The figure shows three views and two pictorial views of one solid part (mm, origin at its lowest corner). Answer the questions. A direction names the side the tool comes from. Round coordinates to 2 decimals unless told otherwise and drop trailing zeros.
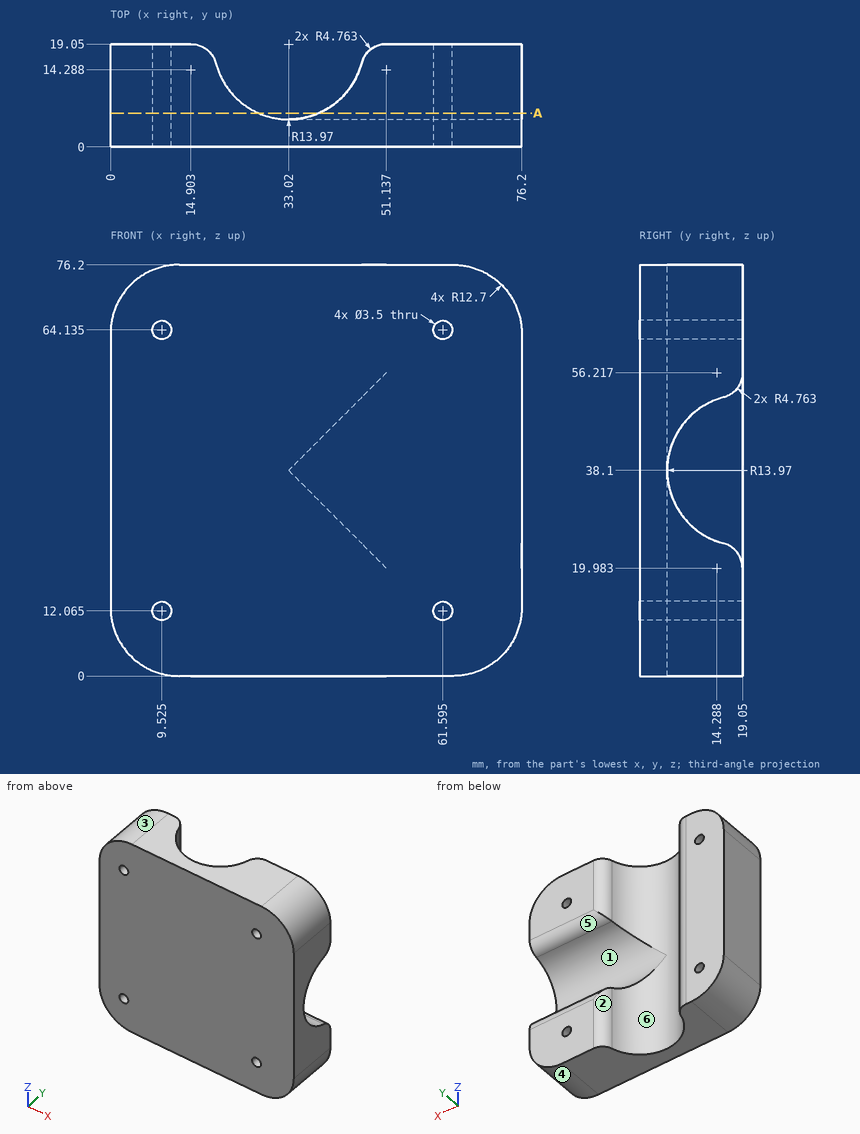
Item 1: Find the intervals of material crossed by line 1 along Z through (x, y) = (63, 17) (1 decimal); line 2 along X through (y, z) = (16, 11) (1 decimal); line 3 along X through (y, z) = (15, 56.5), in increasing order.
Item 2: Find section A-A (y = 6.25). State how many separate pieces and enclosed holes the cut face has, plus the area to 3 significant figures.
Item 3: A tool of negligible diameter and unlimited length cuts with its end or side. For the marked faces 1, 2 and 3, from which of +Z, -Z, +X, -X, +Y, -Y can it reach the whole face along a straight path? Write none if from no direction.
Item 4: Given pin 1 (2 mm diameter, centred on y = 4.5, z = 61, fed in from -X); pin 2 (2 mm diameter, centred on x = 33, z = 64, fed in from +Y), each flat-ended and moving along its own axis, determine where each tip first touches the part or whether it passes through.
Item 5: For a pull along X with two mould halves and no side action, classify the marked faces 4, 5 and 6 as released by +X, released by -X, zero draft, split by the parting line, or undercut.
Model answer:
1. line 1: z = 0 to 11, 13.1 to 23.9, 52.3 to 63.1, 65.2 to 76.2
1. line 2: x = 0.1 to 8.1, 10.9 to 19.3, 46.7 to 60.2, 63 to 76.1
1. line 3: x = 0 to 19.65, 46.39 to 76.2
2. separate pieces: 3
2. enclosed holes: 4
2. area: 4,360 mm2
3. face 1: +X, +Y
3. face 2: +Z, -Z, +Y
3. face 3: +Z, -X, +Y, -Y
4. pin 1: stops at x = 0
4. pin 2: stops at y = 5.12
5. face 4: released by +X
5. face 5: zero draft
5. face 6: undercut
